Autodesk Inventor part; units mm, degrees
ref_plane "YZ Plane" through (0, 0, 0) normal (1, 0, 0) x (0, 1, 0)
ref_plane "XZ Plane" through (0, 0, 0) normal (0, 1, 0) x (-1, 0, 0)
ref_plane "XY Plane" through (0, 0, 0) normal (0, 0, 1) x (1, 0, 0)
sketch "Esboço1" plane through (0, 0, 0) normal (0, 1, 0) x (-1, 0, 0)
  line L0 (-36.0569, -1.2) -> (-1.2, -1.2)
  line L1 (-36.0569, -1.2) -> (-36.0569, -19.2)
  line L2 (-36.0569, -19.2) -> (-20.4684, -19.2)
  arc A0 (-36.0569, -28.2) -> (-20.4684, -19.2) centre (-36.0569, -10.2) ccw
  line L3 (-36.0569, -28.2) -> (-36.0569, -10.2) construction
  line L4 (-20.4684, -19.2) -> (-36.0569, -10.2) construction
  arc A1 (-36.0569, -46.2) -> (-1.2, -19.2) centre (-36.0569, -10.2) ccw
  line L5 (-36.0569, -28.2) -> (-36.0569, -46.2)
  line L6 (-1.2, -1.2) -> (-1.2, -19.2)
  line L7 (0, 0) -> (-37.2569, 0)
  line L8 (-37.2569, 0) -> (-37.2569, -20.4)
  line L9 (-37.2569, -20.4) -> (-22.7077, -20.4)
  arc A2 (-37.2569, -26.9571) -> (-22.7077, -20.4) centre (-36.0569, -10.2) ccw
  line L10 (-37.2569, -26.9571) -> (-37.2569, -47.6526)
  line L11 (0, -19.2) -> (0, 0)
  line L12 (-36.0569, -28.2) -> (-37.2569, -28.2)
  line L13 (-36.0569, -46.2) -> (-37.2569, -46.2)
  line L14 (-36.0569, -1.2) -> (-37.2569, -1.2)
  line L15 (-36.0569, -19.2) -> (-37.2569, -19.2)
  line L16 (-1.2, -19.2) -> (0, -19.2)
  line L17 (-1.2, -1.2) -> (0, -1.2)
  line L18 (-37.2569, -26.9571) -> (-37.2569, -20.4)
  line L19 (0, -20.4) -> (0, -19.2)
  arc A3 (-37.2569, -47.6526) -> (0, -20.4) centre (-36.0569, -10.2) ccw
  point P0 (-28.2626, -19.2)
  point P1 (-18.6284, 0)
  point P2 (8.0774, -19.7542)
  dimension "d19" = 60
  dimension "d21" = 18
  dimension "d22" = 1.2
  dimension "d32" = 1.2
  dimension "d33" = 1.2
extrude "Extrusão2" add sketch "Esboço1" against normal blind 1.2
extrude "Extrusão3" add sketch "Esboço1" along normal blind 9 contours L14 L8 L7 L11 L17 L0 | L2 A0 L12 L10 A2 L9 L8 L15 | L9 A2 L18
extrude "Extrusão4" add sketch "Esboço1" along normal blind 12.6 contours L14 L8 L7 L11 L17 L0 | L16 L19 A3 L10 L13 A1
fillet "Arredondamento2" radius 9 7 edges at (36.6569, 0, -46.2) (14.0114, 0, -38.6605) (0.6, 0, -19.2) (18.6284, 0, -1.2) (36.6569, 0, -28.2) (27.0569, 0, -25.7885) (28.8626, 0, -19.2)
equation "\"Diâmetro_esfera\" = 18"
equation "\"Filamento\" = 0.4"
equation "\"Margem\" = 3 * Filamento"
properties part number "Receptor" material "Plástico PET"
The model under review builds one solid part; all positions refer to its coordinate system, in mm. A direction names the side the tool comes from. Coordinates: 2 decimals unless noted, no trailing zeros. Order: outer loops, then holes, each group sorted by start corner. A loop starts at its lowest first (then second) coordinate and runs counter-clockwise, first axis right, second up. Notation, with made-up numbers: (-25.5, 32.5) -> (24.5, 32.5) arc R20 cw to (24.5, 36.5) -> close; hole circle Ø5 at (-30.75, -21). An arc over 180 degrees is marked (long way). Answer in a Markdown table with one row per item.
(1) The part is to be moulded in two halves that separate along Z. For faces 1 (the flat face through (18, 6, 0)), 2 (the flat face through (19, 12.6, -1)), 3 (the flat face through (31, 9, -23)), 4 (the cylindrical face through (13.75, 10.775, -38.456)), say which applies: +Z half, -Z half, draft (parallel to the pull), parting line (faces both ways), or undercut.
Answers:
| item | result |
|---|---|
| face 1 | +Z half |
| face 2 | draft |
| face 3 | undercut |
| face 4 | undercut |
(2) Machinability: for faces 5 (the cylindrical face through (2.452, 0.885, -14.093)), 6 (the flat face through (0, -0.4, -10.2)), 7 (the flat face through (37, 11, -46.2)), which of the approach directions +Z, -Z, +X, -X, +Y, -Y give a long, thin tool a straight path to every point of the face, cutting with its end or side? Answer none if there is none.
Answers:
| item | result |
|---|---|
| face 5 | +X, -X, +Y |
| face 6 | +Z, -Z, -X, +Y, -Y |
| face 7 | +X, +Y |
(3) Wall thickness on line 1 along Z through (x, y) = (32.5, 1.5); line 2 along Z through (x, y) = (24, 1); line 3 along Z through (x, y) = (7, 5.5): over which ranges is each line inside the solid? List them lowest first.
Answers:
| item | result |
|---|---|
| line 1 | -47.5 to -41.98, -31.94 to -15.18, -5.22 to 0 |
| line 2 | -45.68 to -38.89, -29.64 to -14.32, -6.08 to 0 |
| line 3 | -33.86 to -30.23, -1.91 to 0 |
(4) Consider section D-D (z = -9.5). Write out the cut boundary in (x, y), plus the area to 3 significant figures.
Answers:
| item | result |
|---|---|
| outline | (0, -1.2) -> (37.26, -1.2) -> (37.26, 0.03) -> (0, 0.03) -> close |
| area | 45.7 mm² |
(5) Consider section C-C (y = 6). Write out the cut boundary in (x, z), plus the area to 3 significant figures.
Answers:
| item | result |
|---|---|
| outline | (0, -20.4) arc R37.47 ccw to (37.26, -47.65) -> (37.26, -45.69) -> (36.06, -45.69) arc R35.49 cw to (1.6, -18.69) -> (0, -18.69) -> close; (0, -1.71) -> (37.26, -1.71) -> (37.26, 0) -> (0, 0) -> close; (19.6, -18.69) arc R18.51 ccw to (36.06, -28.71) -> (37.26, -28.71) -> (37.26, -18.69) -> close |
| area | 293 mm² |
(6) Consider section B-B (y = 2.5). Write out the cut boundary in (x, z).
Answers:
| item | result |
|---|---|
| outline | (0, -20.4) arc R37.47 ccw to (37.26, -47.65) -> (37.26, -43.43) -> (36.06, -43.43) arc R33.23 cw to (3.42, -16.43) -> (0, -16.43) -> close; (0, -3.97) -> (37.26, -3.97) -> (37.26, 0) -> (0, 0) -> close; (16.24, -16.43) arc R20.77 ccw to (36.06, -30.97) -> (37.26, -30.97) -> (37.26, -16.43) -> close |
(7) Consider section A-A (y = 9.5). Write out the cut boundary in (x, z), plus the area to 3 significant figures.
Answers:
| item | result |
|---|---|
| outline | (0, -20.4) arc R37.47 ccw to (37.26, -47.65) -> (37.26, -46.2) -> (36.06, -46.2) arc R36 cw to (1.2, -19.2) -> (0, -19.2) -> close; (0, -1.2) -> (37.26, -1.2) -> (37.26, 0) -> (0, 0) -> close |
| area | 118 mm² |
(8) Insertion check: pin 1 (2.5 mm diameter, centred on x = 27.5, z = -24.5, fed in from +Y); pin 2 (3 mm diameter, centred on x = 25, z = -29.5, fed in from +Y); pin 3 (1.5 mm diameter, centred on x = 15, y = 5, fed in from -Z). Each pin has a flat end and moves straight along its axis. Give the tip position at first contact, or say it passes through.
Answers:
| item | result |
|---|---|
| pin 1 | y = 9 |
| pin 2 | y = 2.53 |
| pin 3 | z = -41.69 |
